The drawing under review shows one solid part. Ordinate dimensions are in mm from its lowest x, y, z. A direction names the side the tool comes from. Round coordinates to 2 decimals unless told otherwise and drop trailing zeros. Order: outer loops, then holes, each group sorted by start corner. A loop starts at its lowest first (then second) coordinate and runs counter-clockwise, first axis right, second up. Notation, with made-up numbers: M 63,69.5 L 111,69.5 A18 ccw 111,84.5 Z; hole C 45,81.25 d1. An arc over 180 degrees is marked long. Answer as a JSON object with one key per item and string values. Group by question number.
1. Add section B-B on y = 6. State the section outline as (x, z) points, and give its area (3 significant figures).
2. Add section D-D on z = 3. State the section outline as (x, y) points.
3. To check wall thickness, follow probe 1 along Y at (x, z) = (30, 10.1); probe 2 along X at (y, z) = (67.5, 1.25); probe 3 along Y at (x, z) = (8, 7). State the ranges of each line that lie inside material, in increasing order. Write a range as [from, to].
4. Add section C-C on y = 80. State the section outline as (x, z) points.
5. Clearance check with flat-ended pins moving along their axes: P1, Ø4, axis at x = 11, z = 9, coming from the +Y side; P2, Ø2, axis at x = 17, z = 5, coming from the +Y side; P3, Ø9, axis at x = 8, y = 6, coming from the -Z side; P4, Ø2, axis at x = 54, y = 67, coming from the +Z side. State where each tip first meets the part, or that it passes through.
6. Machinability: for the marked faces 1 and 2, which of the approach directions +Z, -Z, +X, -X, +Y, -Y give a long, thin tool a straight path to every point of the face, cutting with its end or side? Answer none if there is none.
7. Add section A-A on x = 30. State the section outline as (y, z) points, and give its area (3 significant figures).
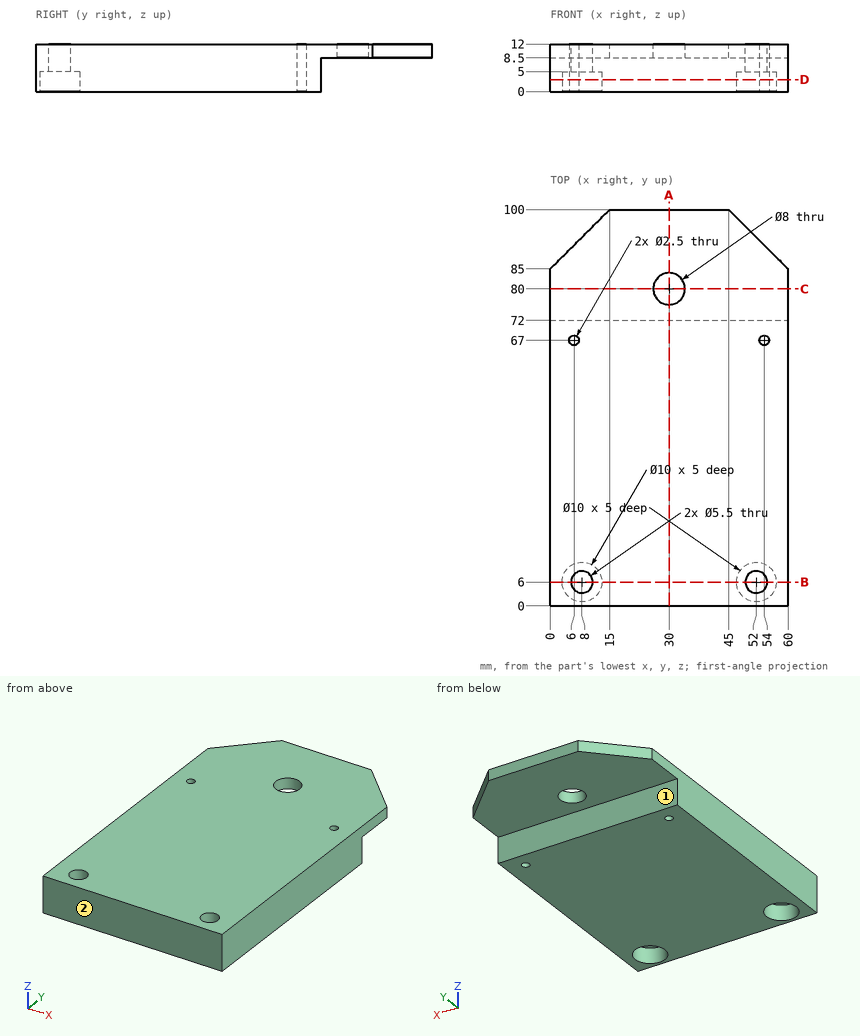
Recorded:
{
 "1": {"outline": "M 0,0 L 3,0 L 3,5 L 5.25,5 L 5.25,12 L 0,12 Z; M 10.75,5 L 13,5 L 13,0 L 47,0 L 47,5 L 49.25,5 L 49.25,12 L 10.75,12 Z; M 54.75,5 L 57,5 L 57,0 L 60,0 L 60,12 L 54.75,12 Z", "area": "543 mm²"},
 "2": {"outline": "M 0,0 L 60,0 L 60,72 L 0,72 Z; hole C 8,6 d10; hole C 6,67 d2.5; hole C 52,6 d10; hole C 54,67 d2.5"},
 "3": {"probe 1": "y = [0, 76], [84, 100]", "probe 2": "x = [0, 4.85], [7.15, 52.85], [55.15, 60]", "probe 3": "y = [0, 3.25], [8.75, 72]"},
 "4": {"outline": "M 0,8.5 L 26,8.5 L 26,12 L 0,12 Z; M 34,8.5 L 60,8.5 L 60,12 L 34,12 Z"},
 "5": {"P1": "stops at y = 98", "P2": "stops at y = 72", "P3": "stops at z = 5", "P4": "passes through"},
 "6": {"face 1": "-Z, +X, -X, +Y", "face 2": "+Z, -Z, +X, -X, -Y"},
 "7": {"outline": "M 0,0 L 72,0 L 72,8.5 L 76,8.5 L 76,12 L 0,12 Z; M 84,8.5 L 100,8.5 L 100,12 L 84,12 Z", "area": "934 mm²"}
}
